Part model, mm, in its own coordinate system. A direction names the side the tool comes from. Round coordinates to 2 decimals unless told otherwise and drop trailing zeros. Loops run counter-clockwise (first coordinate to the right, second up) from the corner with the lowest first, then second, coordinate; pieces in that order, holes last. Notation, with made-up numbers: (55, -9.75) - (69, -9.75) arc R19 ccw to (69, 7.25) - close; hole circle Ø7 at (51, -28). An arc over 180 degrees is marked (long way). Put each result on its own line as item: value.
from build123d import *

# Parameters (mm, degrees)
SKETCH1_R                = 8
SKETCH1_R_2              = 5
BOSS_EXTRUDE1_DEPTH      = 5
SKETCH2_R                = 8
BOSS_EXTRUDE2_DEPTH      = 2
SKETCH3_R                = 2.6
CUT_EXTRUDE1_DEPTH       = 2
CUT_EXTRUDE2_START       = -8
CUT_EXTRUDE2_OUTLINE_W   = 9
CUT_EXTRUDE2_OUTLINE_H   = 18
CUT_EXTRUDE2_DEPTH       = 6.564795928
CUT_EXTRUDE2_START_2     = 1.435204072
CUT_EXTRUDE2_2_OUTLINE_W = 9
CUT_EXTRUDE2_2_OUTLINE_H = 18
CUT_EXTRUDE2_2_DEPTH     = 6.564795928


# Read off the part's stored shape, not the designer's step: Cut-Extrude2
with BuildPart() as part:
    # Sketch1 → Boss-Extrude1 (new body)
    # profile 1 of 7: a face of its own
    with BuildSketch(Plane(origin=(0, 0, 0), x_dir=(1, 0, 0), z_dir=(0, 1, 0))):
        with Locations(Location((0, 0, 0), (0, 0, 270))):
            Circle(SKETCH1_R)
        Circle(SKETCH1_R_2, mode=Mode.SUBTRACT)
    # profile 2 of 7: a face of its own
    with BuildSketch(Plane(origin=(0, 0, 0), x_dir=(1, 0, 0), z_dir=(0, 1, 0))):
        with BuildLine():
            Line((-5, 0), (-2.5, 4.330127019))
            ThreePointArc((-2.5, 4.330127019), (-4.330127019, 2.5), (-5, 0))
        make_face()
    # profile 3 of 7: a face of its own
    with BuildSketch(Plane(origin=(0, 0, 0), x_dir=(1, 0, 0), z_dir=(0, 1, 0))):
        with BuildLine():
            Line((-2.5, -4.330127019), (-5, 0))
            ThreePointArc((-5, 0), (-4.330127019, -2.5), (-2.5, -4.330127019))
        make_face()
    # profile 4 of 7: a face of its own
    with BuildSketch(Plane(origin=(0, 0, 0), x_dir=(1, 0, 0), z_dir=(0, 1, 0))):
        with BuildLine():
            Line((2.5, -4.330127019), (-2.5, -4.330127019))
            ThreePointArc((-2.5, -4.330127019), (0, -5), (2.5, -4.330127019))
        make_face()
    # profile 5 of 7: a face of its own
    with BuildSketch(Plane(origin=(0, 0, 0), x_dir=(1, 0, 0), z_dir=(0, 1, 0))):
        with BuildLine():
            ThreePointArc((2.5, -4.330127019), (4.330127019, -2.5), (5, 0))
            Line((5, 0), (2.5, -4.330127019))
        make_face()
    # profile 6 of 7: a face of its own
    with BuildSketch(Plane(origin=(0, 0, 0), x_dir=(1, 0, 0), z_dir=(0, 1, 0))):
        with BuildLine():
            ThreePointArc((5, 0), (4.330127019, 2.5), (2.5, 4.330127019))
            Line((2.5, 4.330127019), (5, 0))
        make_face()
    # profile 7 of 7: a face of its own
    with BuildSketch(Plane(origin=(0, 0, 0), x_dir=(1, 0, 0), z_dir=(0, 1, 0))):
        with BuildLine():
            ThreePointArc((2.5, 4.330127019), (0, 5), (-2.5, 4.330127019))
            Line((-2.5, 4.330127019), (2.5, 4.330127019))
        make_face()
    extrude(amount=BOSS_EXTRUDE1_DEPTH)

    # Sketch2 → Boss-Extrude2 (add)
    with BuildSketch(Plane(origin=(0, 5, 0), x_dir=(1, 0, 0), z_dir=(0, 1, 0))):
        with Locations(Location((0, 0, 0), (0, 0, 270))):
            Circle(SKETCH2_R)
    extrude(amount=BOSS_EXTRUDE2_DEPTH)

    # Sketch3 → Cut-Extrude1 (cut)
    with BuildSketch(Plane.XZ.offset(-5)):
        with Locations(Location((0, 0, 0), (0, 0, 270))):
            Circle(SKETCH3_R)
    extrude(amount=-CUT_EXTRUDE1_DEPTH, mode=Mode.SUBTRACT)

    # Sketch5 → Revolve1 (revolve)
    with BuildSketch(Plane.XY):
        with BuildLine():
            Line((-8, 0), (-5.5, 0))
            ThreePointArc((-5.5, 0), (-3.889087297, -3.889087297), (0, -5.5))
            Line((0, -5.5), (0, -8))
            ThreePointArc((0, -8), (-5.656854249, -5.656854249), (-8, 0))
        make_face()
    revolve(axis=Axis((0, 5, 0), (0, -1, 0)))

    # Cut-Extrude2 outline → Cut-Extrude2 (cut)
    with BuildSketch(Plane.YZ.offset(CUT_EXTRUDE2_START)):
        with Locations((-4.5, 0)):
            Rectangle(CUT_EXTRUDE2_OUTLINE_W, CUT_EXTRUDE2_OUTLINE_H)
    extrude(amount=CUT_EXTRUDE2_DEPTH, mode=Mode.SUBTRACT)

    # Cut-Extrude2 2 outline → Cut-Extrude2 2 (cut)
    with BuildSketch(Plane.YZ.offset(CUT_EXTRUDE2_START_2)):
        with Locations((-4.5, 0)):
            Rectangle(CUT_EXTRUDE2_2_OUTLINE_W, CUT_EXTRUDE2_2_OUTLINE_H)
    extrude(amount=CUT_EXTRUDE2_2_DEPTH, mode=Mode.SUBTRACT)


solid = part.part
1. Band-saw the part on C-C (x = 0). List the corners of the cut face in (y, z).
A:
outline: (0, -8) - (7, -8) - (7, -2.6) - (5, -2.6) - (5, -4.33) - (0, -4.33) - (0, -5.5) arc R5.5 cw to (0, 5.5) - (0, 4.33) - (5, 4.33) - (5, 2.6) - (7, 2.6) - (7, 8) - (0, 8) arc R8 ccw to start
2. Band-saw the part on A-A (y = 0.25). List the corners of the cut face in (x, z), plus the area to 3 significant figures.
A:
outline: circle Ø16 at (0, 0); hole (-5, 0) - (-2.5, -4.33) - (2.5, -4.33) - (5, 0) - (2.5, 4.33) - (-2.5, 4.33) - close
area: 136 mm²
3. Tool access for faces 4 (the cylindrical face through (0.78, 5.99, -2.48)), 5 (the flat face through (0, 2, -4.33)), 6 (the flat face through (-3.73, 2.46, 2.2)), 7 (the flat face through (-1.435, -6, 0)): list every direction of +Z, -Z, +X, -X, +Y, -Y with a clear straight run to the whole face (end or side of a thin tool).
A:
face 4: +Y
face 5: none
face 6: -Y
face 7: +Z, -Z, -X, -Y
4. Band-saw the part on B-B (z = -0.5). List the corners of the cut face in (x, y), plus the area to 3 significant figures.
A:
outline: (-7.98, 0) - (-4.71, 0) - (-4.71, 5) - (-2.55, 5) - (-2.55, 7) - (-7.98, 7) - close; (-1.44, -7.85) arc R7.98 ccw to (1.44, -7.85) - (1.44, -5.29) arc R5.48 cw to (-1.44, -5.29) - close; (2.55, 5) - (4.71, 5) - (4.71, 0) - (7.98, 0) - (7.98, 7) - (2.55, 7) - close
area: 61.7 mm²
5. Pin check, flat tips, straight feed: P1, Ø1.5, axis at x = 1, y = 2.5, coming from the -Z side; P2, Ø2, axis at x = 6, z = 4, coming from the -Y side; P3, Ø6, axis at y = 4, z = 4.5, coming from the -X side. Stop position of each tip, or through.
A:
P1: stops at z = -8
P2: stops at y = 0
P3: stops at x = -7.86
6. Band-saw the part on D-D (y = -2.75). List the corners of the cut face in (x, z).
A:
outline: (-1.44, -7.37) arc R7.51 ccw to (1.44, -7.37) - (1.44, -4.54) arc R4.76 cw to (-1.44, -4.54) - close; (-1.44, 4.54) arc R4.76 cw to (1.44, 4.54) - (1.44, 7.37) arc R7.51 ccw to (-1.44, 7.37) - close
7. Two-plate mould, pull along X, no slides. Class faces 1 (the flat face through (2, 7, -2)), 2 (the flat face through (1.435, -6, 0)), 3 (the flat face through (0, 2, 4.33)): pulls with the +X half, pulls with the -X half, needs draft (parallel to the pull), parting line crosses it, or undercut.
A:
face 1: needs draft
face 2: pulls with the +X half
face 3: undercut
8. Probe line 1 along X through (y, z) = (6.3, 0); line 2 along Y through (x, z) = (2.25, 2.75); line 3 along Y through (x, z) = (-5, 1.25). List the from-to ranges inside material, lowest first. Write a range as [from, to].
A:
line 1: x = [-8, -2.6], [2.6, 8]
line 2: y = [5, 7]
line 3: y = [0, 7]
